Drawing for the job (mm, zero at the part's lowest x, y, z). A direction names the side the tool comes from. Coordinates: 2 decimals unless noted, no trailing zeros. Order: outer loops, then holes, each group sorted by start corner. A loop starts at its lowest first (then second) coordinate and runs counter-clockwise, first axis right, second up.
1) Tool access for the marked faces 5 and 6: list every direction of +Z, -Z, +X, -X, +Y, -Y with a clear straight run to the whole face (end or side of a thin tool).
2) Cut at D-D (x = 17). List the corners of the cut face in (y, z).
3) Cut at C-C (y = 11). List the corners of the cut face in (x, z).
4) Wall check: L1, parallel to Z at x = 12.5, y = 1.8; L2, parallel to X at y = 18.5, z = 17.75. Give the ranges that are in metal, low to high.
5) Mould opens along Y. For the marked faces 1, 2, 3 and 4 say: +Y half, -Y half, draft (parallel to the pull), parting line (faces both ways), or undercut.
6) Pin check, flat tips, straight feed: pin 1 Ø7 at (y, z) = (11, 7) entering from -X; pin 2 Ø10 at (y, z) = (19, 23) entering from +X; pin 3 Ø8 at (x, z) = (15, 14.5) entering from +Y; pin 4 Ø5 at (x, z) = (12.5, 15) entering from -Y. Stop position of each tip, or through.
7) Cut at B-B (z = 12.25). List the corners of the cut face in (x, y), and give its area (3 significant figures).
8) Cut at A-A (x = 12.5). List the corners of the cut face in (y, z), and give its area (3 significant figures).
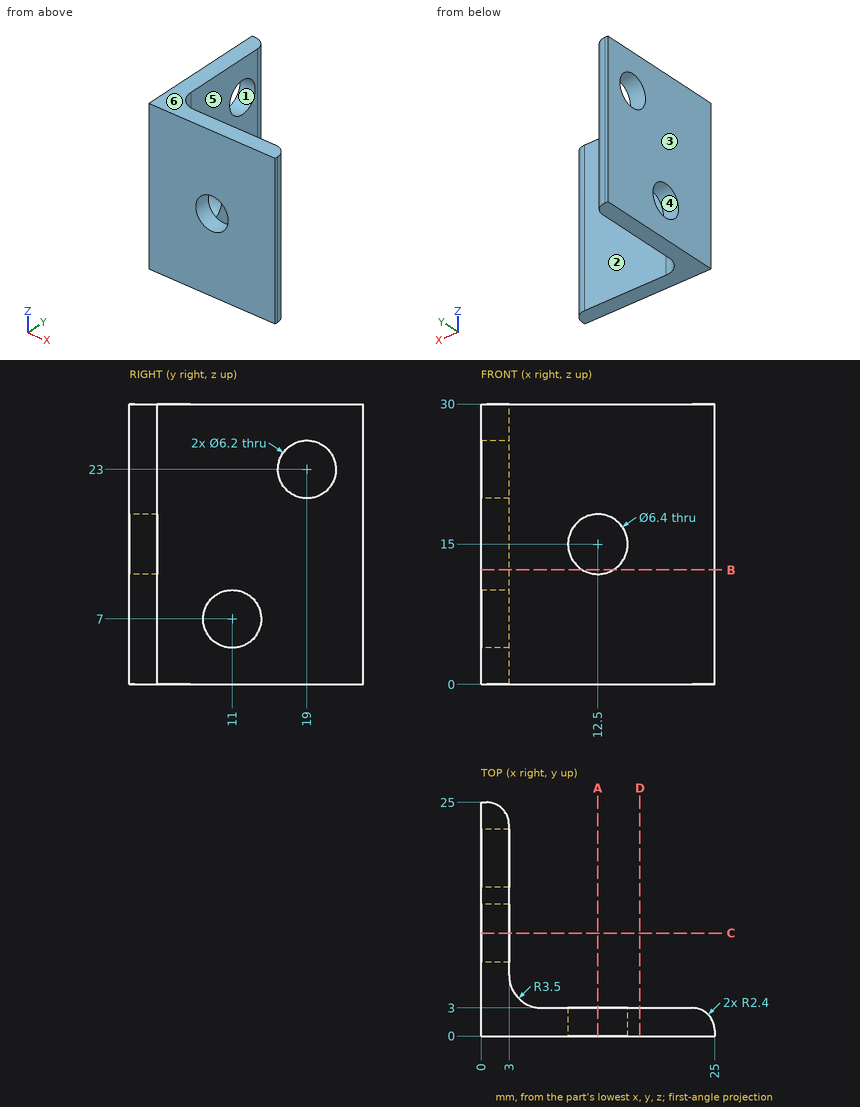
Geometry check:
1. face 5: +Z, -Z, +X, +Y
1. face 6: +Z, +X, -X, +Y, -Y
2. outline: (0, 0) - (3, 0) - (3, 30) - (0, 30) - close
3. outline: (0, 0) - (3, 0) - (3, 3.9) - (0, 3.9) - close; (0, 10.1) - (3, 10.1) - (3, 30) - (0, 30) - close
4. L1: z = 0 to 11.8, 18.2 to 30
4. L2: x = 0 to 3
5. face 1: undercut
5. face 2: +Y half
5. face 3: draft
5. face 4: undercut
6. pin 1: stops at x = 0
6. pin 2: stops at x = 3
6. pin 3: stops at y = 3
6. pin 4: passes through
7. outline: (0, 0) - (10.86, 0) - (10.86, 3) - (6.5, 3) arc R3.5 cw to (3, 6.5) - (3, 22.6) arc R2.4 ccw to (0.6, 25) - (0, 25) - close; (14.14, 0) - (25, 0) - (25, 0.6) arc R2.4 ccw to (22.6, 3) - (14.14, 3) - close
7. area: 131 mm2
8. outline: (0, 0) - (3, 0) - (3, 11.8) - (0, 11.8) - close; (0, 18.2) - (3, 18.2) - (3, 30) - (0, 30) - close
8. area: 70.8 mm2
